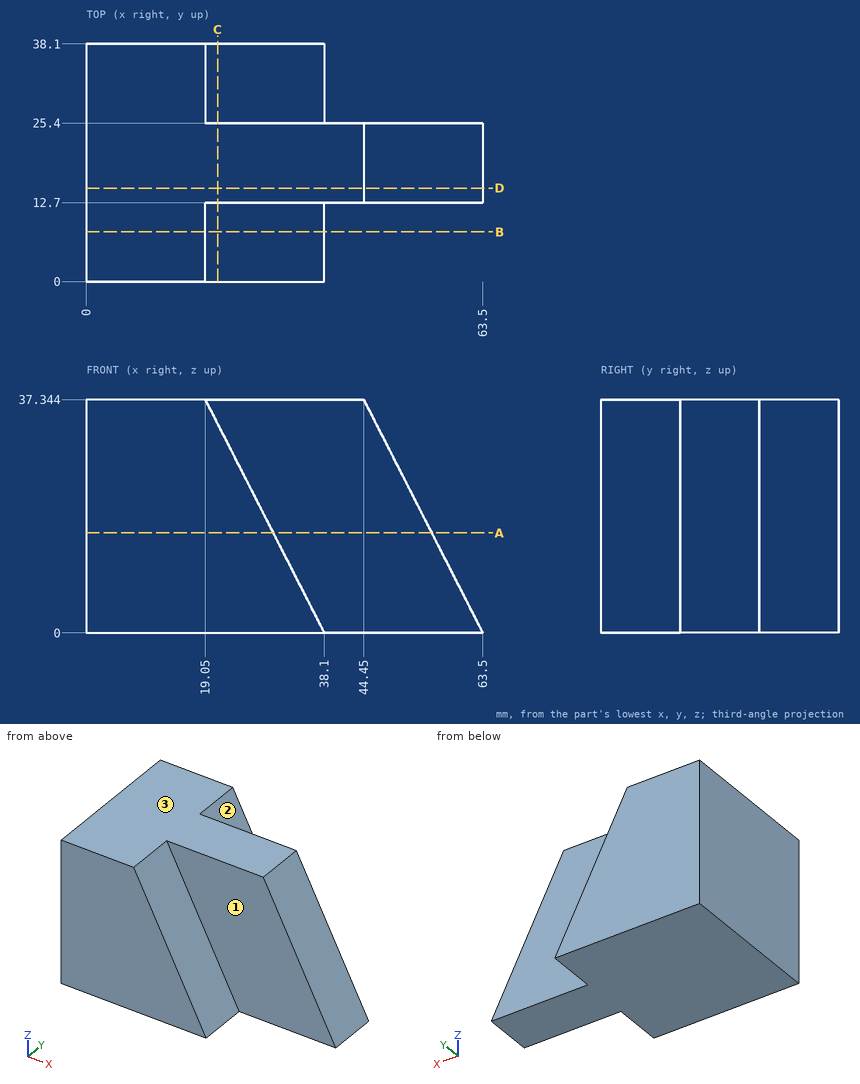
Source: three-view drawing plus pictorial views. Frame: mm from the lowest corner of the part. A direction names the side the tool comes from. Coordinates: 2 decimals unless noted, no trailing zeros. Write each loop counter-clockwise with the first axis right and the second up, starting at its lowest first coordinate (ties: lowest second). Pieces come first, ordered by that corner, then holes. Notation, with made-up numbers: (-24, 65) - (18, 65) arc R14 ccw to (18, 89) - close; hole circle Ø3 at (-14.75, 81). An arc over 180 degrees is marked (long way). Answer as a JSON object with one key per item and string values.
Q1. Material intervals for line 1 (Y direction, x = 43, z = 35.5); line 2 (Z direction, x = 23, y = 11); line 3 (X direction, y = 10, z = 14), sorted ascending. Write a range as [from, to].
Ans:
{"line 1": "y = [12.7, 25.4]", "line 2": "z = [0, 29.6]", "line 3": "x = [0, 30.96]"}
Q2. Set-up query: the marked faces 1, 2 and 3. Return all of +Z, -Z, +X, -X, +Y, -Y with unobstructed straight access to the full face (end or side cutting, diameter ignored); none if empty.
Ans:
{"face 1": "+Z, +X, -Y", "face 2": "+Z, +X, +Y", "face 3": "+Z, +X, -X, +Y, -Y"}
Q3. First-contact query: pin 1 Ø8 at (y, z) = (19, 30.5) entering from +X; pin 2 Ø3 at (x, z) = (54.5, 10.5) entering from -Y; pin 3 Ø12 at (x, z) = (54.5, 11) entering from +Y. Flat tips, straight axial feed; report the tip coordinate or a pass-through.
Ans:
{"pin 1": "stops at x = 49.98", "pin 2": "stops at y = 12.7", "pin 3": "stops at y = 25.4"}
Q4. Section query A-A, the plane z = 16. Output: boundary loops of the cut face in (x, y).
Ans:
{"outline": "(0, 0) - (29.94, 0) - (29.94, 12.7) - (55.34, 12.7) - (55.34, 25.4) - (29.94, 25.4) - (29.94, 38.1) - (0, 38.1) - close"}
Q5. Section query C-C, the plane x = 21. Output: boundary loops of the cut face in (y, z).
Ans:
{"outline": "(0, 0) - (38.1, 0) - (38.1, 33.52) - (25.4, 33.52) - (25.4, 37.34) - (12.7, 37.34) - (12.7, 33.52) - (0, 33.52) - close"}
Q6. Section query D-D, the plane y = 15. Output: boundary loops of the cut face in (x, z).
Ans:
{"outline": "(0, 0) - (63.5, 0) - (44.45, 37.34) - (0, 37.34) - close"}
Q7. Section query B-B, the plane y = 8. Output: boundary loops of the cut face in (x, z).
Ans:
{"outline": "(0, 0) - (38.1, 0) - (19.05, 37.34) - (0, 37.34) - close"}
